Here's how the part is built. I have some questions about the finished solid (model axes, mm). A direction names the side the tool comes from. Give positions to 0.01 mm unless a question says otherwise; leave off trailing zeros. Order: outer loops, then holes, each group sorted by start corner. A loop starts at its lowest first (then second) coordinate and runs counter-clockwise, first axis right, second up. Notation, with made-up numbers: M -23,73 L 36,73 A23 cw 36,84 Z; hole C 27.25,14 d4. An arc over 180 degrees is marked long. Use CSV: the item, a comma, the result in double quotes. Start each with the question number.
```python
from build123d import *

# Parameters (mm, degrees)
SKETCH1_W           = 30
SKETCH1_H           = 33
BOSS_EXTRUDE1_DEPTH = 4
SKETCH2_W           = 30
SKETCH2_H           = 40
BOSS_EXTRUDE2_DEPTH = 4
SKETCH4_W           = 30
SKETCH4_H           = 14
BOSS_EXTRUDE3_DEPTH = 4
BOSS_EXTRUDE4_DEPTH = 3


with BuildPart() as part:
    # Sketch1 → Boss-Extrude1 (new body)
    with BuildSketch(Plane.XY):
        with Locations((15, 16.5)):
            Rectangle(SKETCH1_W, SKETCH1_H)
    extrude(amount=BOSS_EXTRUDE1_DEPTH)

    # Sketch2 → Boss-Extrude2 (add)
    with BuildSketch(Plane(origin=(0, 33, 0), x_dir=(1, 0, 0), z_dir=(0, 1, 0))):
        with Locations((15, -20)):
            Rectangle(SKETCH2_W, SKETCH2_H)
    extrude(amount=BOSS_EXTRUDE2_DEPTH)

    # Sketch4 → Boss-Extrude3 (add)
    with BuildSketch(Plane.XZ):
        with Locations((15, 7)):
            Rectangle(SKETCH4_W, SKETCH4_H)
    extrude(amount=BOSS_EXTRUDE3_DEPTH)

    # Sketch3 → Boss-Extrude4 (add)
    with BuildSketch(Plane.XZ.offset(4)):
        Polygon((7.65, 14), (22.35, 14), (24.85, 34), (5.15, 34), align=None)
    extrude(amount=-BOSS_EXTRUDE4_DEPTH)


solid = part.part
```
Q1. Imagine slicing it at D-D, the plane x = 19. Please give me the cut outline in (y, z), then the cut area to 3 significant figures.
Q2. Imagine slicing it at C-C, the plane x = 5.75. Please give me the cut outline in (y, z), then the cut area to 3 significant figures.
Q3. I need wall thicknesses on line 1 (Y direction, x = 15.5, z = 4.5); line 2 (Y direction, x = 13.5, z = 15.5); line 3 (Y direction, x = 2, z = 29.5). Which ranges of each line are inside material? Lowest first, please. Write a range as [from, to].
Q4. For faces 1 (the face through (23.583, -2.521, 23.86)), 2 (the face through (14.8, -0.6, 14)), 3 (the face through (15, 17, 0)), 4 (the face through (15, 33, 22)), 5 (the face through (6.382, -2.521, 24.14)), which set-ups out of +Z, -Z, +X, -X, +Y, -Y let a thin tool reach every point of the face, with its end or its side?
Q5. For P1, Ø6, axis at x = 5.5, y = 11, coming from the +Z side; P2, Ø1.2, axis at x = 8.5, y = -1.5, coming from the +Z side; P3, Ø10, axis at y = 2.5, z = 26, coming from the -X side, each with a flat end and sliding along its axis, tell me the tip position at first contact or that it passes through.
Q6. Imagine slicing it at A-A, the plane x = 23. Please give me the cut outline in (y, z), then the cut area to 3 significant figures.
Q7. We'd pull the mould along Y, two halves only. Please class faces 6 (the face through (15, -4, 13)), 7 (the face through (15, -3, 34)), 8 (the face through (15, 0, 9)): pulls with the +Y half, pulls with the -Y half, needs draft (parallel to the pull), parting line crosses it, or undercut.
Q8. Imagine slicing it at B-B, the plane z = 22. Please give me the cut outline in (x, y).
Reply:
1,outline,"M -4,0 L 37,0 L 37,40 L 33,40 L 33,4 L 0,4 L 0,14 L -1,14 L -1,34 L -4,34 Z"
1,area,"408 mm^2"
2,outline,"M -4,0 L 37,0 L 37,40 L 33,40 L 33,4 L 0,4 L 0,14 L -4,14 Z; M -4,29.2 L -1,29.2 L -1,34 L -4,34 Z"
2,area,"362 mm^2"
3,line 1,"y = [-4, 0], [33, 37]"
3,line 2,"y = [-4, -1], [33, 37]"
3,line 3,"y = [33, 37]"
4,face 1,"+X, -Y"
4,face 2,"none"
4,face 3,"-Z, +X, -X, +Y, -Y"
4,face 4,"+Z, +X, -X"
4,face 5,"-X, -Y"
5,P1,"stops at z = 4"
5,P2,"stops at z = 34"
5,P3,"stops at x = 5.7"
6,outline,"M -4,0 L 37,0 L 37,40 L 33,40 L 33,4 L 0,4 L 0,14 L -4,14 Z; M -4,19.2 L -1,19.2 L -1,34 L -4,34 Z"
6,area,"392 mm^2"
7,face 6,"pulls with the -Y half"
7,face 7,"needs draft"
7,face 8,"undercut"
8,outline,"M 0,33 L 30,33 L 30,37 L 0,37 Z; M 6.65,-4 L 23.35,-4 L 23.35,-1 L 6.65,-1 Z"
